Part model, mm, in its own coordinate system. Face numbers are marked on the shaded views. Give positions to 0.01 mm unless a question says otherwise; leave off trailing zeros. Write each loop counter-clockwise with the first axis right and the second up, starting at its lowest first coordinate (ties: lowest second). Pieces come first, ordered by that corner, then holes. Notation, with made-up numbers: M 42,81.25 L 62,81.25 A25 cw 62,113.25 Z; hole C -27.5,-7.5 d1. An arc over 180 degrees is marked long. Use CSV: the item, a comma, the result in double quotes. Start each with the question number.
1. Drill centre lines: line 1 along X through (y, z) = (259, 571.5); line 2 along Z through (x, y) = (979, -210). Where is each one in solid material? Low to high. Write a range as from..to.
2. Band-saw the part on B-B, the plane x = 1075.5. List the corners of the cut face in (y, z).
3. Mould opens along Y. For the marked faces 1 and 2 say: pulls with the +Y half, pulls with the -Y half, needs draft (parallel to the pull), parting line crosses it, or undercut.
4. Band-saw the part on A-A, the plane y = -97.5. List the corners of the cut face in (x, z), then the cut area to 3 significant figures.
5. Drop flat-ended pins along their axis: pin 1 Ø3 at (x, z) = (973, 499.5) entering from -Y; pin 2 Ø3 at (x, y) = (1126.5, 91) entering from -Z; pin 3 Ø0.6 at (x, y) = (976.5, -291) entering from -Z; pin 4 Ø1 at (x, y) = (975, 291) entering from +Z. Give the stop position or say it passes through.
6. Band-saw the part on C-C, the plane z = 519. List the corners of the cut face in (x, y), then the cut area to 3 significant figures.
7. Band-saw the part on D-D, the plane x = 997. List the corners of the cut face in (y, z), then the cut area to 3 significant figures.
from build123d import *

# Parameters (mm, degrees)
WYCI_GNI_CIE_CIENKA_CIANKA1_DEPTH      = 400
WYCI_GNI_CIE_CIENKA_CIANKA1_DEPTH_BACK = 400
DODANIE_WYCI_GNI_CIE2_DEPTH            = 2
SZKIC6_W                               = 389.49
SZKIC6_H                               = 5
WYCI_GNI_CIE_CIENKA_CIANKA2_DEPTH      = 1
WYCI_GNI_CIE_CIENKA_CIANKA2_DEPTH_BACK = 1
SZKIC6_2_W                             = 389.49
SZKIC6_2_H                             = 1
WYCI_GNI_CIE_CIENKA_CIANKA3_DEPTH      = 5
WYCI_GNI_CIE_CIENKA_CIANKA3_DEPTH_BACK = 5
SZKIC7_R                               = 2
WYTNIJ_WYCI_GNI_CIE1_DEPTH             = 10
SZKIC9_W                               = 10
SZKIC9_H                               = 2
WYCI_GNI_CIE_CIENKA_CIANKA4_DEPTH      = 10
SZKIC10_R                              = 2
WYTNIJ_WYCI_GNI_CIE2_DEPTH             = 10
SKETCH1_R                              = 4
BOSS_EXTRUDE1_DEPTH                    = 12


with BuildPart() as part:
    # Szkic1 → Wyci_gni_cie-cienka _cianka1 (new, two sides)
    with BuildSketch(Plane(origin=(0, 0, 0), x_dir=(1, 0, 0), z_dir=(0, 1, 0))) as wyci_gni_cie_cienka_cianka1_sk:
        Polygon((956.950680953, -465.228422764), (970.58269303, -477.059346089), (970.58269303, -617.999346089), (1360.07269303, -617.999346089), (1360.07269303, -618.499346089), (970.08269303, -618.499346089), (970.08269303, -477.287451692), (956.622954545, -465.606040827), align=None)
    extrude(amount=WYCI_GNI_CIE_CIENKA_CIANKA1_DEPTH)
    extrude(wyci_gni_cie_cienka_cianka1_sk.sketch, amount=-WYCI_GNI_CIE_CIENKA_CIANKA1_DEPTH_BACK)

    # Ci_cie powierzchni_1
    split(bisect_by=Plane(origin=(90.906039695, 464.075841363, 0), x_dir=(-0.9813493581662637, 0.19223276834780917, 0), z_dir=(0.19223276834780917, 0.9813493581662637, 0)), keep=Keep.BOTTOM)

    # Ci_cie powierzchni_2
    split(bisect_by=Plane(origin=(90.906039695, -464.075841363, 0), x_dir=(-0.9813493581662637, -0.19223276834780917, 0), z_dir=(-0.19223276834780917, 0.9813493581662637, 0)), keep=Keep.TOP)

    # Szkic4 → Dodanie-wyci_gni_cie2 (add)
    with BuildSketch(Plane(origin=(90.906039695, -464.075841363, 0), x_dir=(-0.9813493581662637, -0.19223276834780914, 0), z_dir=(0.19223276834780914, -0.9813493581662637, 0))):
        with BuildLine():
            Line((-896.394995334, -587.669895838), (-896.394995334, -567.646267832))
            ThreePointArc((-896.394995334, -567.646267832), (-907.43844862, -577.658081835), (-896.394995334, -587.669895838))
        make_face()
    dodanie_wyci_gni_cie2 = extrude(amount=-DODANIE_WYCI_GNI_CIE2_DEPTH)

    # Szkic6 → Wyci_gni_cie-cienka _cianka2 (add, two sides)
    with BuildSketch(Plane(origin=(0, 0, 0), x_dir=(1, 0, 0), z_dir=(0, 1, 0))) as wyci_gni_cie_cienka_cianka2_sk:
        with Locations((1165.32769303, -615.499346089)):
            Rectangle(SZKIC6_W, SZKIC6_H)
    extrude(amount=WYCI_GNI_CIE_CIENKA_CIANKA2_DEPTH)
    extrude(wyci_gni_cie_cienka_cianka2_sk.sketch, amount=-WYCI_GNI_CIE_CIENKA_CIANKA2_DEPTH_BACK)

    # Szkic6_2 → Wyci_gni_cie-cienka _cianka3 (add, two sides)
    with BuildSketch(Plane(origin=(0, 0, 0), x_dir=(1, 0, 0), z_dir=(0, 1, 0))) as wyci_gni_cie_cienka_cianka3_sk:
        with Locations((1165.32769303, -617.499346089)):
            Rectangle(SZKIC6_2_W, SZKIC6_2_H)
    extrude(amount=WYCI_GNI_CIE_CIENKA_CIANKA3_DEPTH)
    extrude(wyci_gni_cie_cienka_cianka3_sk.sketch, amount=-WYCI_GNI_CIE_CIENKA_CIANKA3_DEPTH_BACK)

    # Szkic7 → Wytnij-wyci_gni_cie1 (cut)
    with BuildSketch(Plane(origin=(90.521574159, -462.113142647, 0), x_dir=(0.9813493581662637, 0.19223276834780917, 0), z_dir=(-0.19223276834780914, 0.9813493581662636, 0))):
        with Locations(Location((901.117736464, -577.428231407, 0), (0, 0, 180))):
            Circle(SZKIC7_R)
    wytnij_wyci_gni_cie1 = extrude(amount=-WYTNIJ_WYCI_GNI_CIE1_DEPTH, mode=Mode.SUBTRACT)

    # Lustro1: Dodanie-wyci_gni_cie2, Wytnij-wyci_gni_cie1 across plane
    add(dodanie_wyci_gni_cie2.mirror(Plane.ZX))
    add(wytnij_wyci_gni_cie1.mirror(Plane.ZX), mode=Mode.SUBTRACT)

    # Szkic9 → Wyci_gni_cie-cienka _cianka4 (add)
    with BuildSketch(Plane(origin=(970.58269303, 0, 0), x_dir=(0, 0, -1), z_dir=(1, 0, 0))):
        with Locations((-497.999346089, -290.759349877)):
            Rectangle(SZKIC9_W, SZKIC9_H)
    wyci_gni_cie_cienka_cianka4 = extrude(amount=WYCI_GNI_CIE_CIENKA_CIANKA4_DEPTH)

    # Szkic10 → Wytnij-wyci_gni_cie2 (cut)
    with BuildSketch(Plane(origin=(0, -289.759349877, 0), x_dir=(1, 0, 0), z_dir=(0, 1, 0))):
        with Locations(Location((975.58269303, -497.999346089, 0), (0, 0, 270))):
            Circle(SZKIC10_R)
    wytnij_wyci_gni_cie2 = extrude(amount=-WYTNIJ_WYCI_GNI_CIE2_DEPTH, mode=Mode.SUBTRACT)

    # Sketch1 → Boss-Extrude1 (add)
    with BuildSketch(Plane(origin=(0, 0, 617.999346089), x_dir=(-1, 0, 0), z_dir=(0, 0, -1))):
        with Locations(Location((-1233.504191335, -222.034079566, 0), (0, 0, 180))):
            Circle(SKETCH1_R)
    boss_extrude1 = extrude(amount=BOSS_EXTRUDE1_DEPTH)

    # Lustro2: Wyci_gni_cie-cienka _cianka4, Wytnij-wyci_gni_cie2, Boss-Extrude1 across plane
    add(wyci_gni_cie_cienka_cianka4.mirror(Plane.ZX))
    add(wytnij_wyci_gni_cie2.mirror(Plane.ZX), mode=Mode.SUBTRACT)
    add(boss_extrude1.mirror(Plane.ZX))


solid = part.part
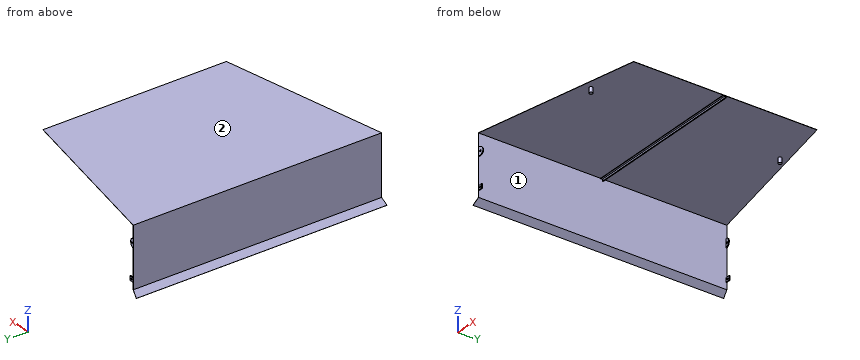
Output:
1,line 1,"x = 970.08..970.58"
1,line 2,"z = 618..618.5"
2,outline,"M -271.21,618 L -5,618 L -5,617 L -1,617 L -1,613 L 1,613 L 1,617 L 5,617 L 5,618 L 271.21,618 L 271.21,618.5 L -271.21,618.5 Z"
3,face 1,"undercut"
3,face 2,"needs draft"
4,outline,"M 956.62,465.61 L 956.95,465.23 L 970.58,477.06 L 970.58,618 L 1360.07,618 L 1360.07,618.5 L 970.08,618.5 L 970.08,477.29 Z"
4,area,"274 mm²"
5,pin 1,"stops at y = -291.76"
5,pin 2,"stops at z = 618"
5,pin 3,"stops at z = 493"
5,pin 4,"stops at z = 618.5"
6,outline,"M 970.08,-291.86 L 970.58,-291.76 L 970.58,291.76 L 970.08,291.86 Z"
6,area,"292 mm²"
7,outline,"M -286.58,618 L -5,618 L -5,617 L -1,617 L -1,613 L 1,613 L 1,617 L 5,617 L 5,618 L 286.58,618 L 286.58,618.5 L -286.58,618.5 Z"
7,area,"305 mm²"
